The figure shows three views and two pictorial views of one solid part (mm, origin at its lowest corner). Answer the questions. A direction names the side the tool comes from. Coordinates: 2 decimals unless noted, no trailing zeros. Order: outer loops, then holes, each group sorted by start corner. A loop starts at its lowest first (then second) coordinate and runs counter-clockwise, first axis right, second up. Notation, with made-up numbers: (20.5, 13.5) - (57.5, 13.5) arc R20 ccw to (57.5, 52.5) - close; hole circle Ø8 at (-13.5, 19). An arc over 180 degrees is marked (long way). Use one line per item in the form item = value.
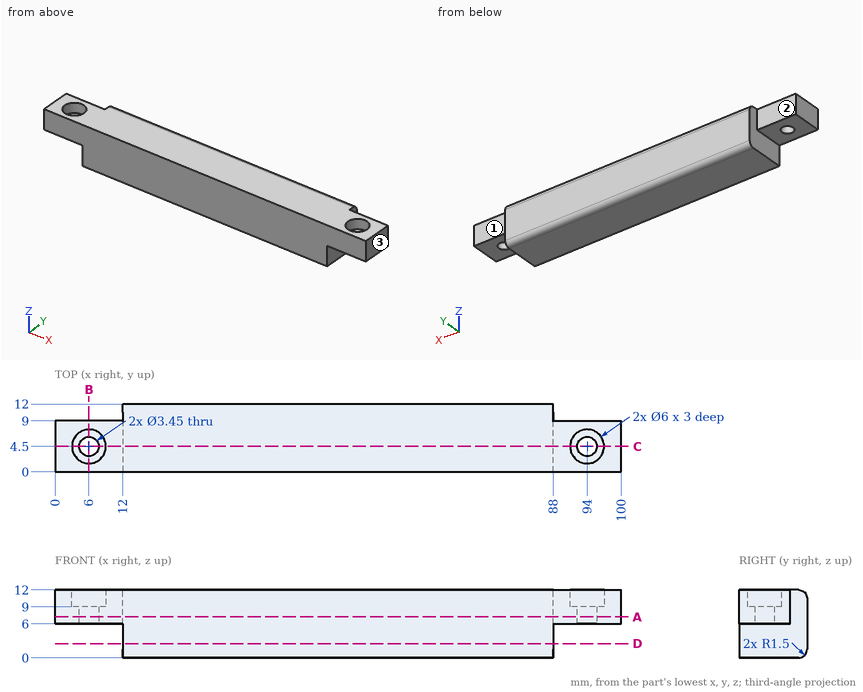
(1) Section C-C, the plane y = 4.5 is taken. Write down the section's boundary in (x, z) (3 decimals).
Answer list:
outline = (0, 6) - (4.275, 6) - (4.275, 9) - (3, 9) - (3, 12) - (0, 12) - close; (7.725, 6) - (12, 6) - (12, 0) - (88, 0) - (88, 6) - (92.275, 6) - (92.275, 9) - (91, 9) - (91, 12) - (9, 12) - (9, 9) - (7.725, 9) - close; (95.725, 6) - (100, 6) - (100, 12) - (97, 12) - (97, 9) - (95.725, 9) - close
(2) Section B-B, the plane x = 6 is taken. Write down the section's boundary in (y, z) (3 decimals), then the cut area to 4 significant figures.
Answer list:
outline = (0, 6) - (2.775, 6) - (2.775, 9) - (1.5, 9) - (1.5, 12) - (0, 12) - close; (6.225, 6) - (9, 6) - (9, 12) - (7.5, 12) - (7.5, 9) - (6.225, 9) - close
area = 25.65 mm2
(3) Which of the six approach directions +Z, -Z, +X, -X, +Y, -Y give full straight-line access (tool end or side, diameter ignored) to the marked faces 1, 2 and 3?
Answer list:
face_1 = +Z, -Z, +X, +Y
face_2 = +Z, -Z, -X, +Y
face_3 = +Z, -Z, +X, +Y, -Y
(4) Given pin 1 Ø6.5 at (x, z) = (94, 9.5) entering from +Y; pin 2 Ø4.5 at (x, y) = (6, 4.5) entering from -Z; pin 3 Ø3 at (x, y) = (6.5, 5) entering from +Z; pin 4 Ø3 at (x, y) = (94, 4.5) entering from +Z, each flat-ended and moving along its own axis, determine where each tip first touches the part or whether it passes through.
Answer list:
pin_1 = 9
pin_2 = 6
pin_3 = 9
pin_4 = through
(5) Section A-A, the plane z = 7.25 is taken. Write down the section's boundary in (x, y) (3 decimals), then the cut area to 3 significant figures.
Answer list:
outline = (0, 0) - (100, 0) - (100, 9) - (88, 9) - (88, 12) - (12, 12) - (12, 9) - (0, 9) - close; hole circle Ø3.45 at (6, 4.5); hole circle Ø3.45 at (94, 4.5)
area = 1,110 mm2
(6) Straight lines are drawn through the part: L1, parallel to Y at x = 6, z = 8.2 (3 decimals); L2, parallel to Y at x = 6, z = 11.1; L3, parallel to Z at x = 28, y = 10.75. For each, find the intervals that lie inside material, in ascending order.
Answer list:
L1 = 0 to 2.775, 6.225 to 9
L2 = 0 to 1.5, 7.5 to 9
L3 = 0.02 to 11.98
(7) Section D-D, the plane z = 2.5 is taken. Write down the section's boundary in (x, y).
Answer list:
outline = (12, 0) - (88, 0) - (88, 12) - (12, 12) - close
